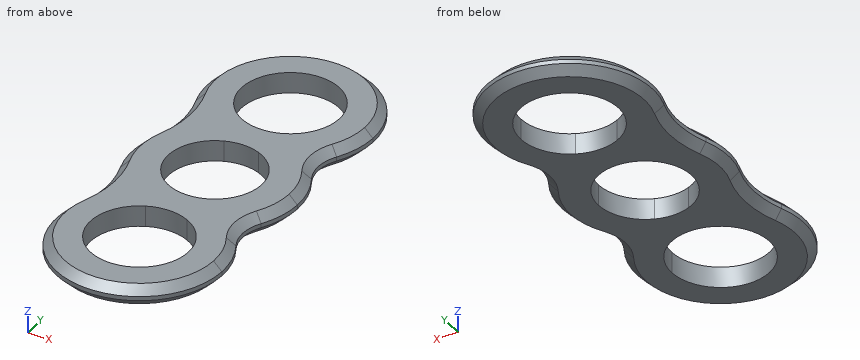
```python
from build123d import *

# Parameters (mm, degrees)
F1_DEPTH = 5
F2_R     = 10
F3_R     = 25
F4_SIZE  = 2
F5_SIZE  = 2


with BuildPart() as f1:
    # F0 (on Top) → F1 (new body)
    with BuildSketch(Plane.XY):
        with BuildLine():
            ThreePointArc((-4.137504636, -10.4615273926), (-11.25, 0), (-4.137504636, 10.4615273926))
            ThreePointArc((-4.137504636, 10.4615273926), (-8.9686549041, 12.1525425178), (-13.2123684763, 15.0144370273))
            ThreePointArc((-13.2123684763, 15.0144370273), (-20, 0), (-13.2123684763, -15.0144370273))
            ThreePointArc((-13.2123684763, -15.0144370273), (-8.9686549041, -12.1525425178), (-4.137504636, -10.4615273926))
        make_face()
        with BuildLine():
            ThreePointArc((4.137504636, 10.4615273926), (9.303478574, 6.3251708611), (11.25, 0))
            ThreePointArc((11.25, 0), (9.303478574, -6.3251708611), (4.137504636, -10.4615273926))
            ThreePointArc((4.137504636, -10.4615273926), (8.9686549041, -12.1525425178), (13.2123684763, -15.0144370273))
            ThreePointArc((13.2123684763, -15.0144370273), (18.2242608839, -8.2387083476), (20, 0))
            ThreePointArc((20, 0), (18.2242608839, 8.2387083476), (13.2123684763, 15.0144370273))
            ThreePointArc((13.2123684763, 15.0144370273), (8.9686549041, 12.1525425178), (4.137504636, 10.4615273926))
        make_face()
        with BuildLine():
            ThreePointArc((-4.137504636, 10.4615273926), (0, 11.25), (4.137504636, 10.4615273926))
            ThreePointArc((4.137504636, 10.4615273926), (8.9686549041, 12.1525425178), (13.2123684763, 15.0144370273))
            ThreePointArc((13.2123684763, 15.0144370273), (9.3655087913, 17.6716508872), (5.0068447736, 19.3631481277))
            ThreePointArc((5.0068447736, 19.3631481277), (0, 18.2464208238), (-5.0068447736, 19.3631481277))
            ThreePointArc((-5.0068447736, 19.3631481277), (-9.3655087913, 17.6716508872), (-13.2123684763, 15.0144370273))
            ThreePointArc((-13.2123684763, 15.0144370273), (-8.9686549041, 12.1525425178), (-4.137504636, 10.4615273926))
        make_face()
        with BuildLine():
            ThreePointArc((13.2123684763, -15.0144370273), (8.9686549041, -12.1525425178), (4.137504636, -10.4615273926))
            ThreePointArc((4.137504636, -10.4615273926), (0, -11.25), (-4.137504636, -10.4615273926))
            ThreePointArc((-4.137504636, -10.4615273926), (-8.9686549041, -12.1525425178), (-13.2123684763, -15.0144370273))
            ThreePointArc((-13.2123684763, -15.0144370273), (-9.3655087913, -17.6716508872), (-5.0068447736, -19.3631481277))
            ThreePointArc((-5.0068447736, -19.3631481277), (0, -18.2464208238), (5.0068447736, -19.3631481277))
            ThreePointArc((5.0068447736, -19.3631481277), (9.3655087913, -17.6716508872), (13.2123684763, -15.0144370273))
        make_face()
        with BuildLine():
            ThreePointArc((5.0068447736, 19.3631481277), (9.3655087913, 17.6716508872), (13.2123684763, 15.0144370273))
            ThreePointArc((13.2123684763, 15.0144370273), (18.2242608839, 21.790165707), (20, 30.0288740546))
            ThreePointArc((20, 30.0288740546), (-8.2387083476, 48.2531349384), (-13.2123684763, 15.0144370273))
            ThreePointArc((-13.2123684763, 15.0144370273), (-9.3655087913, 17.6716508872), (-5.0068447736, 19.3631481277))
            ThreePointArc((-5.0068447736, 19.3631481277), (-6.3179620827, 39.9742025688), (11.7824532307, 30.0288740546))
            ThreePointArc((11.7824532307, 30.0288740546), (9.9453285142, 23.7109119719), (5.0068447736, 19.3631481277))
        make_face()
        with BuildLine():
            ThreePointArc((20, -30.0288740546), (18.2242608839, -21.790165707), (13.2123684763, -15.0144370273))
            ThreePointArc((13.2123684763, -15.0144370273), (9.3655087913, -17.6716508872), (5.0068447736, -19.3631481277))
            ThreePointArc((5.0068447736, -19.3631481277), (9.9453285142, -23.7109119719), (11.7824532307, -30.0288740546))
            ThreePointArc((11.7824532307, -30.0288740546), (-6.3179620827, -39.9742025688), (-5.0068447736, -19.3631481277))
            ThreePointArc((-5.0068447736, -19.3631481277), (-9.3655087913, -17.6716508872), (-13.2123684763, -15.0144370273))
            ThreePointArc((-13.2123684763, -15.0144370273), (-8.2387083476, -48.2531349384), (20, -30.0288740546))
        make_face()
    extrude(amount=F1_DEPTH)

    # F2
    f2_edges = [f1.edges().sort_by_distance(p)[0] for p in [
        (13.212368, -15.014437, 2.5),
        (13.212368, 15.014437, 2.5),
    ]]
    fillet(f2_edges, radius=F2_R)

    # F3
    f3_edges = [f1.edges().sort_by_distance(p)[0] for p in [
        (-13.212368, -15.014437, 2.5),
        (-13.212368, 15.014437, 2.5),
    ]]
    fillet(f3_edges, radius=F3_R)

    # F4
    f4_edges = [f1.edges().sort_by_distance(p)[0] for p in [
        (1.83718, -49.944315, 5),
        (-17.4213, -15.014437, 5),
        (-20, 0, 5),
        (-17.4213, 15.014437, 5),
        (1.83718, 49.944315, 5),
        (15.972422, -15.014437, 5),
        (20, 0, 5),
        (15.972422, 15.014437, 5),
    ]]
    chamfer(f4_edges, length=F4_SIZE)

    # F5
    f5_edges = [f1.edges().sort_by_distance(p)[0] for p in [
        (1.83718, -49.944315, 0),
    ]]
    chamfer(f5_edges, length=F5_SIZE)


solid = f1.part
```
Could you check a few things on this model? Use its own coordinates, in mm. Coordinates: 2 decimals unless noted, no trailing zeros. Loops run counter-clockwise (first coordinate to the right, second up) from the corner with the lowest first, then second, coordinate; pieces in that order, holes last.
1) Imagine slicing it at B-B (x = 6). State how many separate pieces and enclosed holes the cut face has, and give its area (3 significant figures).
Reported:
separate pieces: 4
enclosed holes: 0
area: 185 mm2
2) Please list where these lines run through material, in increasing order: line 1 along Y through (x, z) = (-0.5, 2.9); line 2 along Y through (x, z) = (17, 0.85); line 3 along X through (y, z) = (26, 0.6).
Reported:
line 1: y = -50.02 to -41.8, -18.26 to -11.24, 11.24 to 18.26, 41.8 to 50.02
line 2: y = -38.17 to -21.89, -8.14 to 8.14, 21.89 to 38.17
line 3: x = -18.16 to -11.07, 11.07 to 18.16
3) Imagine slicing it at A-A (x = 0). List the corners of the cut face in (y, z) for me.
Reported:
outline: (-50.03, 2) - (-48.03, 0) - (-41.81, 0) - (-41.81, 5) - (-48.03, 5) - (-50.03, 3) - close; (-18.25, 0) - (-11.25, 0) - (-11.25, 5) - (-18.25, 5) - close; (11.25, 0) - (18.25, 0) - (18.25, 5) - (11.25, 5) - close; (41.81, 0) - (48.03, 0) - (50.03, 2) - (50.03, 3) - (48.03, 5) - (41.81, 5) - close
4) Will these pins go through, and if not, where does the flat tip stop? pin 1 Ø1 at (y, z) = (-17.5, 3) entering from -X; pin 2 Ø1 at (x, z) = (-1.5, 2.5) entering from +Y.
Reported:
pin 1: stops at x = -17.6
pin 2: stops at y = 50
